Check sheet for the modelled part. Datum: model origin and axes. Units: mm. Face numbers are marked on the shaded views. A direction names the side the tool comes from. Give positions to 0.01 mm unless a question says otherwise; leave off trailing zeros. Write each loop counter-clockwise with the first axis right and the second up, starting at its lowest first coordinate (ties: lowest second). Pieces come first, ordered by that corner, then holes. Notation, with made-up numbers: (54.5, -34.75) -> (71.5, -34.75) arc R19 cw to (71.5, 1.25) -> close; hole circle Ø10 at (-24, 24.5). An arc over 180 degrees is marked (long way). Use a Markdown table: item, result. Add a question column.
1. Cross-section at A-A (x = 10). Enter the section's corners in (y, z), then the cut area to 3 significant figures.
2. Cross-section at D-D (x = 39). Enter the section's corners in (y, z), then the cut area to 3 significant figures.
3. Release check for a two-part mould opening along X. For the marked faces 3, 4, 5 and 6 record: released by +X, released by -X, zero draft, split by the parting line, or undercut.
4. Scan lines: probe 1 along Y at (x, z) = (10, 12.6); probe 2 along X at (y, z) = (7.5, 4.75); probe 3 along Y at (x, z) = (11, 8.5). Record each from-to range of solid material in increasing order. Write a range as [from, to].
5. Gauge pin test, flat ends, axial feed: P1, Ø2.5, axis at x = -10, y = 5, coming from the -Z side; P2, Ø6, axis at x = -40.5, y = 4.5, coming from the -Z side; P3, Ø4, axis at x = 10, y = 5, coming from the -Z side; P4, Ø3, axis at x = -57.5, y = 1.5, coming from the -Z side. Record the tip position at first contact, or that the pin passes through.
6. Cross-section at C-C (x = -40). Enter the section's corners in (y, z), then the cut area to 3 significant figures.
7. Cross-section at B-B (y = 5). Count the separate pieces of the cut face and the enclosed holes in it, then the cut area to 3 significant figures.
8. Set-up check for the marked faces 1 and 2: record each of +Z, -Z, +X, -X, +Y, -Y from which the full face is reachable in a straight line by a thin tool's end or side.
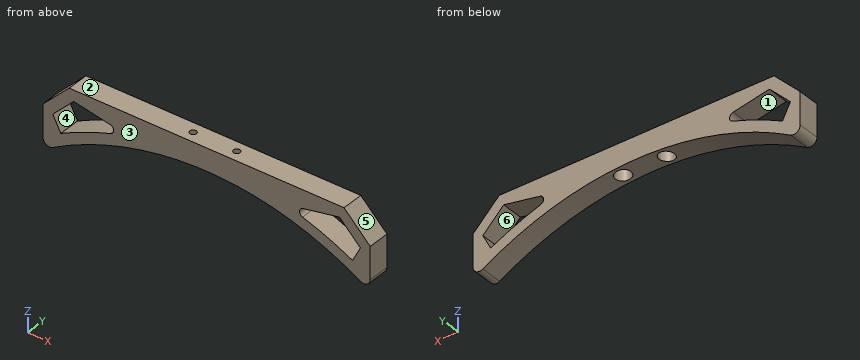
from build123d import *

# Parameters (mm, degrees)
EXTRUDE_1_DEPTH     = 10
CHAMFER_1_SIZE      = 15
FILLET_1_R          = 3
SKETCH_2_R          = 1.5
CUT_EXTRUDE_2_DEPTH = 78.661122835
SKETCH_4_R          = 3.5
CUT_EXTRUDE_3_DEPTH = 10
CUT_EXTRUDE_4_DEPTH = 78.661122848
FILLET_2_R          = 2
SKETCH_6_W          = 150
SKETCH_6_H          = 5.98
CUT_EXTRUDE_5_DEPTH = 78.661122848


with BuildPart() as part:
    # 草图1 → 凸台-拉伸1 (new body)
    with BuildSketch(Plane(origin=(0, 0, 0), x_dir=(1, 0, 0), z_dir=(0, 1, 0))):
        with BuildLine():
            Line((-75, -17.5), (75, -17.5))
            Line((75, -17.5), (75, 17.5))
            ThreePointArc((75, 17.5), (0, -4.284095825), (-75, 17.5))
            Line((-75, 17.5), (-75, -17.5))
        make_face()
    extrude(amount=EXTRUDE_1_DEPTH)

    # 倒角1
    chamfer_1_edges = [part.edges().sort_by_distance(p)[0] for p in [
        (75, 5, 17.5),
        (-75, 5, 17.5),
    ]]
    chamfer(chamfer_1_edges, length=CHAMFER_1_SIZE)

    # 圆角1
    fillet_1_edges = [part.edges().sort_by_distance(p)[0] for p in [
        (75, 5, -17.5),
        (-75, 5, -17.5),
    ]]
    fillet(fillet_1_edges, radius=FILLET_1_R)

    # 草图2 → 切除-拉伸2 (cut, through all)
    with BuildSketch(Plane.XY):
        with Locations(Location((10, 5, 0), (0, 0, 180))):
            Circle(SKETCH_2_R)
        with Locations(Location((-10, 5, 0), (0, 0, 180))):
            Circle(SKETCH_2_R)
    extrude(amount=CUT_EXTRUDE_2_DEPTH, mode=Mode.SUBTRACT)

    # 草图4 → 切除-拉伸3 (cut)
    with BuildSketch(Plane.XY):
        with Locations(Location((10, 5, 0), (0, 0, 180))):
            Circle(SKETCH_4_R)
        with Locations(Location((-10, 5, 0), (0, 0, 180))):
            Circle(SKETCH_4_R)
    extrude(amount=CUT_EXTRUDE_3_DEPTH, mode=Mode.SUBTRACT)

    # 草图5 → 切除-拉伸4 (cut, through all)
    with BuildSketch(Plane.XZ):
        with BuildLine():
            ThreePointArc((-36, 4.744054532), (-51.772161826, -0.273505866), (-66.86977855, -7.055759932))
            Line((-66.86977855, -7.055759932), (-70.5, -0.071067812))
            Line((-70.5, -0.071067812), (-60.928932188, 9.5))
            Line((-60.928932188, 9.5), (-36, 4.744054532))
        make_face()
        with BuildLine():
            Line((60.928932188, 9.5), (36, 4.744054532))
            ThreePointArc((36, 4.744054532), (51.772161826, -0.273505866), (66.86977855, -7.055759932))
            Line((66.86977855, -7.055759932), (70.5, -0.071067812))
            Line((70.5, -0.071067812), (60.928932188, 9.5))
        make_face()
    extrude(amount=-CUT_EXTRUDE_4_DEPTH, mode=Mode.SUBTRACT)

    # 圆角2
    fillet_2_edges = [part.edges().sort_by_distance(p)[0] for p in [
        (-36, 5, 4.744054532),
        (36, 5, 4.744054532),
    ]]
    fillet(fillet_2_edges, radius=FILLET_2_R)

    # 草图6 → 切除-拉伸5 (cut, through all)
    with BuildSketch(Plane.XZ):
        with Locations((0, 17.5)):
            Rectangle(SKETCH_6_W, SKETCH_6_H)
    extrude(amount=-CUT_EXTRUDE_5_DEPTH, mode=Mode.SUBTRACT)


solid = part.part
Worked answers:
| question | item | result |
|---|---|---|
| 1 | outline | (0, 3.93) -> (1.5, 3.93) -> (1.5, 10) -> (3.5, 10) -> (3.5, 14.51) -> (0, 14.51) -> close; (6.5, 10) -> (8.5, 10) -> (8.5, 3.93) -> (10, 3.93) -> (10, 14.51) -> (6.5, 14.51) -> close |
| 1 | area | 49.8 mm² |
| 2 | outline | (0, -1.26) -> (10, -1.26) -> (10, 14.51) -> (0, 14.51) -> close |
| 2 | area | 158 mm² |
| 3 | face 3 | zero draft |
| 3 | face 4 | undercut |
| 3 | face 5 | released by +X |
| 3 | face 6 | undercut |
| 4 | probe 1 | y = [0, 3.5], [6.5, 10] |
| 4 | probe 2 | x = [-72.75, -65.68], [-42.65, -12.45], [-7.55, 7.55], [12.45, 42.65], [65.68, 72.75] |
| 4 | probe 3 | y = [0, 1.65], [8.35, 10] |
| 5 | P1 | passes through |
| 5 | P2 | stops at z = -2.65 |
| 5 | P3 | stops at z = 10 |
| 5 | P4 | stops at z = -8.76 |
| 6 | outline | (0, -1.55) -> (10, -1.55) -> (10, 14.51) -> (0, 14.51) -> close |
| 6 | area | 161 mm² |
| 7 | separate pieces | 3 |
| 7 | enclosed holes | 2 |
| 7 | area | 1,840 mm² |
| 8 | face 1 | +Y, -Y |
| 8 | face 2 | +Z, +X, -X, +Y, -Y |
